The listing builds one solid part. Answer for the finished solid, in the listing's coordinates (mm). A direction names the side the tool comes from. Round coordinates to 2 decimals unless told otherwise and drop trailing zeros. Loops run counter-clockwise (first coordinate to the right, second up) from the corner with the lowest first, then second, coordinate; pieces in that order, holes last. Notation, with made-up numbers: M 69,-19 L 80,-19 A15 ccw 80,-4 Z; hole C -33,41.5 d6. An arc over 180 degrees is marked long. Answer as a JSON object with one key per item and string values.
Autodesk Inventor part; units mm, degrees
ref_plane "YZ Plane" through (0, 0, 0) normal (1, 0, 0) x (0, 1, 0)
ref_plane "XZ Plane" through (0, 0, 0) normal (0, 1, 0) x (-1, 0, 0)
ref_plane "XY Plane" through (0, 0, 0) normal (0, 0, 1) x (1, 0, 0)
sketch "Boceto1" plane through (0, 0, 0) normal (0, 1, 0) x (-1, 0, 0)
  line L0 (-41, 50) -> (41, 50)
  line L1 (45, 46) -> (45, -46)
  line L2 (41, -50) -> (-41, -50)
  line L3 (-45, -46) -> (-45, 46)
  arc A0 (41, -50) -> (45, -46) centre (41, -46) ccw
  arc A1 (45, 46) -> (41, 50) centre (41, 46) ccw
  arc A2 (-41, 50) -> (-45, 46) centre (-41, 46) ccw
  arc A3 (-45, -46) -> (-41, -50) centre (-41, -46) ccw
  line L4 (43.8284, -48.8284) -> (48.8284, -48.8284) construction
  circle A4 centre (40.2929, -45.2929) radius 4
  circle A5 centre (40.2929, 45.2929) radius 4
  circle A6 centre (-40.2929, 45.2929) radius 4
  circle A7 centre (-40.2929, -45.2929) radius 4
  point P0 (0, 0)
extrude "Extrusión1" add sketch "Boceto1" along normal blind 50
sketch "Boceto2" plane through (0, 50, 0) normal (0, 1, 0) x (1, 0, 0)
  circle A0 centre (0, 0) radius 25
  dimension "d19" = 50
extrude "Extrusión2" add sketch "Boceto2" along normal blind 50
sketch "Boceto3" plane through (0, 100, 0) normal (0, 1, 0) x (1, 0, 0)
  circle A0 centre (0, 0) radius 20
  dimension "d22" = 40
extrude "Extrusión3" cut sketch "Boceto3" against normal blind 30
thread "Rosca1"
fillet "Empalme1" radius 2 1 edges at (-25, 100, 0)
properties part number "Pieza No.1 Lj"
Item 1: Straight lines are drawn through the part: line 1 (X direction, y = 45.5, z = -43); line 2 (Y direction, x = 31.5, z = -27); line 3 (Y direction, x = 2, z = 18.5). For each, find the intervals that lie inside material, in ascending order.
Values follow:
{"line 1": "-45 to -43.57, -37.02 to 37.02, 43.57 to 45", "line 2": "0 to 50", "line 3": "0 to 70"}
Item 2: Which of the six approach directions +Z, -Z, +X, -X, +Y, -Y give full straight-line access (tool end or side, diameter ignored) to faces 1 (the face through (1, 25, 50)), 2 (the face through (11, 50, 23))?
Values follow:
{"face 1": "+Z, +X, -X, +Y, -Y", "face 2": "+Y"}
Item 3: The part is cut by section A-A (z = 43.5). Give the vertices of the cut face in (x, y).
Values follow:
{"outline": "M -45,0 L -43.87,0 L -43.87,50 L -45,50 Z; M -36.72,0 L 36.72,0 L 36.72,50 L -36.72,50 Z; M 43.87,0 L 45,0 L 45,50 L 43.87,50 Z"}
Item 4: Determine the mould class of faces 3 (the face through (-37.345, 24.65, -47.996)), 4 (the face through (-7, 100, -19)), 5 (the face through (-43.797, 24.65, 48.859)), 6 (the face through (23.846, 73.664, 7.509)) for opening direction Z: released by +Z, released by -Z, zero draft, split by the parting line, or undercut.
Values follow:
{"face 3": "undercut", "face 4": "zero draft", "face 5": "released by +Z", "face 6": "split by the parting line"}
Item 5: The part is cut by section C-C (y = 37.5). Give the vertices of the cut face in (x, z).
Values follow:
{"outline": "M -45,-46 A4 ccw -41,-50 L 41,-50 A4 ccw 45,-46 L 45,46 A4 ccw 41,50 L -41,50 A4 ccw -45,46 Z; hole C -40.29,-45.29 d8; hole C -40.29,45.29 d8; hole C 40.29,-45.29 d8; hole C 40.29,45.29 d8"}
Item 6: The part is cut by section B-B (x = 39.5). Give the vertices of the cut face in (y, z), then the cut area to 3 significant figures.
Values follow:
{"outline": "M 0,-50 L 50,-50 L 50,-49.21 L 0,-49.21 Z; M 0,-41.37 L 50,-41.37 L 50,41.37 L 0,41.37 Z; M 0,49.21 L 50,49.21 L 50,50 L 0,50 Z", "area": "4,220 mm^2"}
Item 7: The part is cut by section D-D (z = 0). Give the vertices of the cut face in (x, y), then the cut area to 3 significant figures.
Values follow:
{"outline": "M -45,0 L 45,0 L 45,50 L 25,50 L 25,98 A2 ccw 23,100 L 20,100 L 20,70 L -20,70 L -20,100 L -23,100 A2 ccw -25,98 L -25,50 L -45,50 Z", "area": "5,800 mm^2"}
Item 8: Flat-ended cylindrical pins translate along their axes: P1, Ø10, axis at y = 88.5, z = -18, coming from the -X side; P2, Ø1.5, axis at x = 30.5, z = 18, coming from the +Y side; P3, Ø2, axis at x = 7, y = 71.5, coming from the -Z side. Find the tip coordinate at first contact, or state that the pin passes through.
Values follow:
{"P1": "x = -21.35", "P2": "y = 50", "P3": "z = -24.27"}
